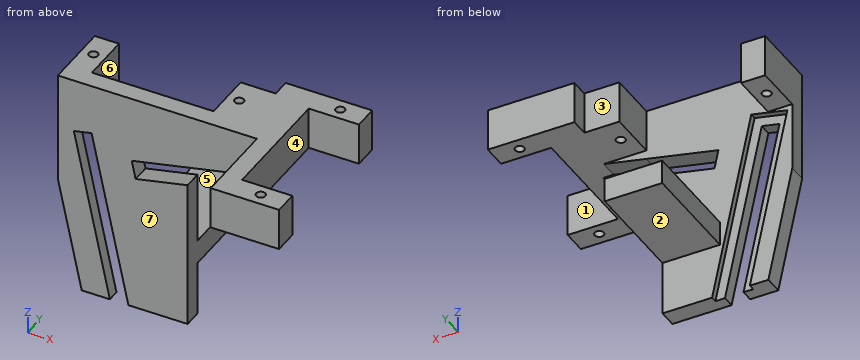
from build123d import *

# Parameters (mm, degrees)
SKETCH1_R               = 0.75
BOSS_EXTRUDE1_DEPTH     = 7
SKETCH9_W               = 32.9
SKETCH9_H               = 14
CUT_EXTRUDE1_DEPTH      = 53.894990311
SKETCH10_W              = 24.1
SKETCH10_H              = 3
BOSS_EXTRUDE2_DEPTH     = 30
CUT_EXTRUDE2_DEPTH      = 57.059254365
CUT_EXTRUDE3_DEPTH      = 57.059254365
CUT_EXTRUDE4_DEPTH      = 1
CUT_EXTRUDE5_DEPTH      = 57.059254365
BOSS_EXTRUDE4_START     = 4
BOSS_EXTRUDE4_OUTLINE_W = 19.373526859
BOSS_EXTRUDE4_OUTLINE_H = 3
BOSS_EXTRUDE4_DEPTH     = 2.47789315
SKETCH21_W              = 25.330744156
SKETCH21_H              = 3
BOSS_EXTRUDE7_DEPTH     = 4
BOSS_EXTRUDE8_START     = 14
BOSS_EXTRUDE8_DEPTH     = 3
CUT_EXTRUDE6_REACH      = 66.171
SKETCH23_W              = 6.651649707
SKETCH23_H              = 3
SKETCH24_W              = 9.5
SKETCH24_H              = 4
BOSS_EXTRUDE9_DEPTH     = 17.5


with BuildPart() as part:
    # Sketch1 → Boss-Extrude1 (new body)
    with BuildSketch(Plane.XY):
        Polygon((0, 0), (0, 25.2), (4, 25.2), (4, 17), (24.1, 17), (24.1, 25.2), (29.9, 25.2), (29.9, 28.2), (44.2, 28.2), (44.2, 24.2), (35.9, 24.2), (35.9, 4), (44.2, 4), (44.2, 0), align=None)
        with Locations((2, 21.1)):
            Circle(SKETCH1_R, mode=Mode.SUBTRACT)
        with Locations((26.1, 21.1)):
            Circle(SKETCH1_R, mode=Mode.SUBTRACT)
        with Locations((40.05, 26.15)):
            Circle(SKETCH1_R, mode=Mode.SUBTRACT)
        with Locations((40.05, 2.05)):
            Circle(SKETCH1_R, mode=Mode.SUBTRACT)
    extrude(amount=BOSS_EXTRUDE1_DEPTH)

    # Sketch9 → Cut-Extrude1 (cut, through all)
    with BuildSketch(Plane.XY.offset(7)):
        with Locations((16.45, 7)):
            Rectangle(SKETCH9_W, SKETCH9_H)
    extrude(amount=-CUT_EXTRUDE1_DEPTH, mode=Mode.SUBTRACT)

    # Sketch10 → Boss-Extrude2 (add)
    with BuildSketch(Plane(origin=(0, 0, 0), x_dir=(-1, 0, 0), z_dir=(0, 0, -1))):
        with Locations((-12.05, 15.5)):
            Rectangle(SKETCH10_W, SKETCH10_H)
    extrude(amount=BOSS_EXTRUDE2_DEPTH)

    # Sketch11 → Cut-Extrude2 (cut, through all)
    with BuildSketch(Plane(origin=(0, 17, 0), x_dir=(1, 0, 0), z_dir=(0, 1, 0))):
        Polygon((8.6, 30), (2.648416273, 2), (5.582859075, 1.376264928), (11.667021785, 30), align=None)
    extrude(amount=-CUT_EXTRUDE2_DEPTH, mode=Mode.SUBTRACT)

    # Sketch12 → Cut-Extrude3 (cut, through all)
    with BuildSketch(Plane(origin=(0, 17, 0), x_dir=(1, 0, 0), z_dir=(0, 1, 0))):
        Polygon((12.20677635, 4.027982726), (24.1, 1.5), (24.1, 4.669255844), (12.851302592, 7.060240288), align=None)
    extrude(amount=-CUT_EXTRUDE3_DEPTH, mode=Mode.SUBTRACT)

    # Sketch14 → Cut-Extrude4 (cut)
    with BuildSketch(Plane(origin=(0, 17, 0), x_dir=(1, 0, 0), z_dir=(0, 1, 0))):
        Polygon((7.015372078, 30), (0.810024371, 0.80613434), (6.776724736, -0.462126974), (13.251649707, 30), align=None)
    extrude(amount=-CUT_EXTRUDE4_DEPTH, mode=Mode.SUBTRACT)

    # Sketch15 → Cut-Extrude5 (cut, through all)
    with BuildSketch(Plane(origin=(0, 17, 0), x_dir=(1, 0, 0), z_dir=(0, 1, 0))):
        Polygon((3.948350293, 30), (0, 11.424472327), (0, 30), align=None)
    extrude(amount=-CUT_EXTRUDE5_DEPTH, mode=Mode.SUBTRACT)

    # Boss-Extrude4: read off the stored shape, not the designer's step
    # Boss-Extrude4 outline → Boss-Extrude4 (add)
    with BuildSketch(Plane(origin=(0, 0, 0), x_dir=(0.9781476007338054, 0, 0.20791169081776006), z_dir=(0.2079116908177601, 0, -0.9781476007338055)).offset(BOSS_EXTRUDE4_START)):
        with Locations((20.78932773, -15.5)):
            Rectangle(BOSS_EXTRUDE4_OUTLINE_W, BOSS_EXTRUDE4_OUTLINE_H)
    extrude(amount=BOSS_EXTRUDE4_DEPTH)

    # Sketch21 → Boss-Extrude7 (add)
    with BuildSketch(Plane(origin=(24.1, 0, 0), x_dir=(0, 0, -1), z_dir=(1, 0, 0))):
        with Locations((17.334627922, 15.5)):
            Rectangle(SKETCH21_W, SKETCH21_H)
    extrude(amount=BOSS_EXTRUDE7_DEPTH)

    # Boss-Extrude8: read off the stored shape, not the designer's step
    # Boss-Extrude8 outline → Boss-Extrude8 (add)
    with BuildSketch(Plane(origin=(0, 0, 0), x_dir=(1, 0, 0), z_dir=(0, 1, 0)).offset(BOSS_EXTRUDE8_START)):
        Polygon((24.1, 4.669255844), (28.1, 3.819029597), (28.1, 4.669255844), align=None)
    extrude(amount=BOSS_EXTRUDE8_DEPTH)

    # Cut-Extrude6: up to this plane
    cut_extrude6_end = Plane(origin=(1.991355959, 0, -9.368593205), z_dir=(0.20791169081775973, 0, -0.9781476007338056))
    # Sketch23 → Cut-Extrude6 (cut, up to the surface)
    with BuildSketch(Plane(origin=(0, 0, -30), x_dir=(-1, 0, 0), z_dir=(0, 0, -1)), mode=Mode.PRIVATE) as cut_extrude6_sk1:
        with Locations((-24.774175146, 15.5)):
            Rectangle(SKETCH23_W, SKETCH23_H)
    cut_extrude6_tool1 = split(extrude(cut_extrude6_sk1.sketch, amount=-CUT_EXTRUDE6_REACH, mode=Mode.PRIVATE), bisect_by=cut_extrude6_end, keep=Keep.BOTH, mode=Mode.PRIVATE)
    add(cut_extrude6_tool1.solids().sort_by_distance((24.774175, 15.5, -30))[0], mode=Mode.SUBTRACT)

    # Sketch24 → Boss-Extrude9 (add)
    with BuildSketch(Plane(origin=(0, 17, 0), x_dir=(1, 0, 0), z_dir=(0, 1, 0))):
        with Locations((16.698350293, 19)):
            Rectangle(SKETCH24_W, SKETCH24_H)
    extrude(amount=BOSS_EXTRUDE9_DEPTH)


solid = part.part
Read the model definition and answer for the solid it produces. Units are mm, in the model's axes. Face numbers are marked on the shaded views. A direction names the side the tool comes from. Round coordinates to 2 decimals unless told otherwise and drop trailing zeros. Order: outer loops, then holes, each group sorted by start corner. A loop starts at its lowest first (then second) coordinate and runs counter-clockwise, first axis right, second up. Notation, with made-up numbers: (9.5, 84.25) - (42.5, 84.25) arc R16 ccw to (42.5, 98.25) - close; hole circle Ø10 at (13, 6). An arc over 180 degrees is marked (long way). Use one line per item in the form item = value. Start each with the question number.
(1) Find the intervals of material crossed by line 1 along Y through (x, z) = (40.05, 5.5); line 2 along X through (y, z) = (21, 3); line 3 along X through (y, z) = (2, 4), in increasing order. Write a range as from..to.
(2) The part is cut by section A-A (y = 2.05). Give the vertices of the cut face in (x, z), then the cut area to 3 significant figures.
(3) The part is cut by section C-C (z = 2.5). Give the vertices of the cut face in (x, y).
(4) The part is cut by section D-D (y = 21.1). Give the vertices of the cut face in (x, z).
(5) Determine the mould class of the marked faces 1, 2 and 3 for opening direction Y: +Y half, -Y half, draft (parallel to the pull), parting line (faces both ways), or undercut.
(6) The part is cut by section B-B (x = 40.05). Give the vertices of the cut face in (y, z), then the cut area to 3 significant figures.
(7) Flat-ended cylindrical pins translate along their axes: pin 1 Ø1.2 at (x, z) = (2.5, 4.5) entering from +Y; pin 2 Ø5 at (x, y) = (7.5, 20) entering from +Z; pin 3 Ø1.5 at (y, z) = (25, -16.5) entering from +X; pin 4 Ø10 at (x, y) = (30.5, 23) entering from -Z. Find the tip coordinate at first contact, or state that the pin passes through.
(8) For the marked faces 4, 5, 6 and 7, determine the directions among +Z, -Z, +X, -X, +Y, -Y from which every point of the face is accessible in a straight line to the end or side of a thin tool.
Checked values:
q1.line_1 = 0..1.3, 2.8..4, 24.2..25.4, 26.9..28.2
q1.line_2 = 0..1.26, 2.74..4, 24.1..25.36, 26.84..35.9
q1.line_3 = 32.9..39.3, 40.8..44.2
q2.outline = (32.9, 0) - (39.3, 0) - (39.3, 7) - (32.9, 7) - close; (40.8, 0) - (44.2, 0) - (44.2, 7) - (40.8, 7) - close
q2.area = 68.6 mm^2
q3.outline = (0, 14) - (32.9, 14) - (32.9, 0) - (44.2, 0) - (44.2, 4) - (35.9, 4) - (35.9, 24.2) - (44.2, 24.2) - (44.2, 28.2) - (29.9, 28.2) - (29.9, 25.2) - (24.1, 25.2) - (24.1, 17) - (4, 17) - (4, 25.2) - (0, 25.2) - close; hole circle Ø1.5 at (2, 21.1); hole circle Ø1.5 at (26.1, 21.1); hole circle Ø1.5 at (40.05, 2.05); hole circle Ø1.5 at (40.05, 26.15)
q4.outline = (0, 0) - (1.25, 0) - (1.25, 7) - (0, 7) - close; (2.75, 0) - (4, 0) - (4, 7) - (2.75, 7) - close; (11.95, -21) - (21.45, -21) - (21.45, -17) - (11.95, -17) - close; (24.1, 0) - (25.35, 0) - (25.35, 7) - (24.1, 7) - close; (26.85, 0) - (35.9, 0) - (35.9, 7) - (26.85, 7) - close
q5.face_1 = undercut
q5.face_2 = draft
q5.face_3 = +Y half
q6.outline = (0, 0) - (1.3, 0) - (1.3, 7) - (0, 7) - close; (2.8, 0) - (4, 0) - (4, 7) - (2.8, 7) - close; (24.2, 0) - (25.4, 0) - (25.4, 7) - (24.2, 7) - close; (26.9, 0) - (28.2, 0) - (28.2, 7) - (26.9, 7) - close
q6.area = 35.0 mm^2
q7.pin_1 = 25.2
q7.pin_2 = through
q7.pin_3 = 21.45
q7.pin_4 = 0
q8.face_4 = +Z, -Z, +X
q8.face_5 = +Z, +X, -X, +Y
q8.face_6 = +Z, -Z, +Y
q8.face_7 = +Z, -Z, -X, -Y
